from build123d import *
from OCP.BRepFilletAPI import BRepFilletAPI_MakeChamfer

# Parameters (mm, degrees)
SKETCH1_W           = 40
SKETCH1_H           = 30
BOSS_EXTRUDE1_DEPTH = 6
SKETCH2_R           = 1.5
CUT_EXTRUDE1_DEPTH  = 6
FILLET1_R           = 4
SKETCH3_W           = 21
SKETCH3_H           = 21
CUT_EXTRUDE2_DEPTH  = 4
SKETCH6_W           = 5
SKETCH6_H           = 5
CUT_EXTRUDE3_DEPTH  = 2
SKETCH7_W           = 7
SKETCH7_H           = 7
SKETCH7_W_2         = 5
SKETCH7_H_2         = 5
BOSS_EXTRUDE2_DEPTH = 4
CHAMFER1_SIZE       = 4
CHAMFER1_SIZE2      = 6.92820323
CHAMFER2_SIZE       = 5
CHAMFER2_SIZE2      = 2.886751346


with BuildPart() as part:
    # Sketch1 → Boss-Extrude1 (new body)
    with BuildSketch(Plane(origin=(0, 0, 0), x_dir=(1, 0, 0), z_dir=(0, 1, 0))):
        with Locations((20, 15)):
            Rectangle(SKETCH1_W, SKETCH1_H)
    extrude(amount=BOSS_EXTRUDE1_DEPTH)

    # Sketch2 → Cut-Extrude1 (cut)
    with BuildSketch(Plane(origin=(0, 6, 0), x_dir=(1, 0, 0), z_dir=(0, 1, 0))):
        with Locations(Location((5, 5, 0), (0, 0, 270))):
            Circle(SKETCH2_R)
        with Locations(Location((5, 25, 0), (0, 0, 90))):
            Circle(SKETCH2_R)
        with Locations(Location((35, 5, 0), (0, 0, 90))):
            Circle(SKETCH2_R)
        with Locations(Location((35, 25, 0), (0, 0, 270))):
            Circle(SKETCH2_R)
    extrude(amount=-CUT_EXTRUDE1_DEPTH, mode=Mode.SUBTRACT)

    # Fillet1
    fillet1_edges = [part.edges().sort_by_distance(p)[0] for p in [
        (0, 3, -30),
        (40, 3, -30),
        (40, 3, 0),
        (0, 3, 0),
    ]]
    fillet(fillet1_edges, radius=FILLET1_R)

    # Sketch3 → Cut-Extrude2 (cut)
    with BuildSketch(Plane(origin=(0, 6, 0), x_dir=(1, 0, 0), z_dir=(0, 1, 0))):
        with Locations((20, 15)):
            Rectangle(SKETCH3_W, SKETCH3_H)
    extrude(amount=-CUT_EXTRUDE2_DEPTH, mode=Mode.SUBTRACT)

    # Sketch6 → Cut-Extrude3 (cut)
    with BuildSketch(Plane(origin=(0, 2, 0), x_dir=(1, 0, 0), z_dir=(0, 1, 0))):
        with Locations((20, 16)):
            Rectangle(SKETCH6_W, SKETCH6_H)
    extrude(amount=-CUT_EXTRUDE3_DEPTH, mode=Mode.SUBTRACT)

    # Sketch7 → Boss-Extrude2 (add)
    with BuildSketch(Plane(origin=(0, 2, 0), x_dir=(1, 0, 0), z_dir=(0, 1, 0))):
        with Locations((20, 16)):
            Rectangle(SKETCH7_W, SKETCH7_H)
        with Locations((20, 16)):
            Rectangle(SKETCH7_W_2, SKETCH7_H_2, mode=Mode.SUBTRACT)
    extrude(amount=BOSS_EXTRUDE2_DEPTH)

    # Chamfer1: one chamfer whose edges measure the first distance from different faces: ONE call of the kernel's chamfer builder (chamfer() names one face for all edges)
    chamfer1_edges_1 = [part.edges().sort_by_distance(p)[0] for p in [
        (20, 0, -13.5),
    ]]
    chamfer1_side_1 = [part.faces().sort_by_distance(p)[0] for p in [
        (20, 3, -13.5),
    ]]
    chamfer1_edges_2 = [part.edges().sort_by_distance(p)[0] for p in [
        (22.5, 0, -16),
    ]]
    chamfer1_side_2 = [part.faces().sort_by_distance(p)[0] for p in [
        (22.5, 3, -16),
    ]]
    chamfer1_edges_3 = [part.edges().sort_by_distance(p)[0] for p in [
        (20, 0, -18.5),
    ]]
    chamfer1_side_3 = [part.faces().sort_by_distance(p)[0] for p in [
        (20, 3, -18.5),
    ]]
    chamfer1_edges_4 = [part.edges().sort_by_distance(p)[0] for p in [
        (17.5, 0, -16),
    ]]
    chamfer1_side_4 = [part.faces().sort_by_distance(p)[0] for p in [
        (17.5, 3, -16),
    ]]
    chamfer1 = BRepFilletAPI_MakeChamfer(part.part.solid().wrapped)
    for e in chamfer1_edges_1:
        chamfer1.Add(CHAMFER1_SIZE, CHAMFER1_SIZE2, e.wrapped, chamfer1_side_1[0].wrapped)  # the first distance lies on this face
    for e in chamfer1_edges_2:
        chamfer1.Add(CHAMFER1_SIZE, CHAMFER1_SIZE2, e.wrapped, chamfer1_side_2[0].wrapped)  # the first distance lies on this face
    for e in chamfer1_edges_3:
        chamfer1.Add(CHAMFER1_SIZE, CHAMFER1_SIZE2, e.wrapped, chamfer1_side_3[0].wrapped)  # the first distance lies on this face
    for e in chamfer1_edges_4:
        chamfer1.Add(CHAMFER1_SIZE, CHAMFER1_SIZE2, e.wrapped, chamfer1_side_4[0].wrapped)  # the first distance lies on this face
    add(Compound.cast(chamfer1.Shape()), mode=Mode.REPLACE)

    # Chamfer2
    chamfer2_edges = [part.edges().sort_by_distance(p)[0] for p in [
        (16.5, 2, -16),
        (20, 2, -12.5),
        (23.5, 2, -16),
        (20, 2, -19.5),
    ]]
    chamfer2_side = [part.faces().sort_by_distance(p)[0] for p in [
        (20, 2, -4.796984848),
    ]]
    chamfer(chamfer2_edges, length=CHAMFER2_SIZE, length2=CHAMFER2_SIZE2, reference=chamfer2_side[0])


solid = part.part
Model file for the job. Use its own axes, mm. A direction names the side the tool comes from. Coordinates: 2 decimals unless noted, no trailing zeros. Order: outer loops, then holes, each group sorted by start corner. A loop starts at its lowest first (then second) coordinate and runs counter-clockwise, first axis right, second up. Notation, with made-up numbers: (73.25, 65) -> (104.25, 65) arc R21 ccw to (104.25, 85) -> close; hole circle Ø8 at (81.25, 4.25). An arc over 180 degrees is marked (long way). Return JSON: item names as keys, results as strings. Group by question number.
Item 1: Pull direction X, two halves, no side cores. Call faces 5 (the flat face through (20, 0, -5)), 6 (the flat face through (26.78, 1.53, -15.87)), 7 (the cylindrical face through (38.797, 3.042, -1.141)), 8 (the flat face through (20, 4, -25.5)): pulls with the +X half, pulls with the -X half, needs draft (parallel to the pull), parting line crosses it, or undercut.
Item 2: Tool access for faces 1 (the flat face through (20, 3, -30)), 2 (the flat face through (30.5, 4, -15)), 3 (the flat face through (19.87, 1.53, -9.22)), 4 (the flat face through (20, 5, -18.5)): list every direction of +Z, -Z, +X, -X, +Y, -Y with a clear straight run to the whole face (end or side of a thin tool).
Item 3: Saw through at B-B on x = 20. Write the cut outline in (y, z), then the cut area to 3 significant figures.
Item 4: Wall check: line 1 along X through (y, z) = (2.8, -25); line 2 along X through (y, z) = (1.5, -5); line 3 along Z through (x, y) = (11, 4). Give the ranges that are in metal, low to high. Write a range as [from, to].
Item 5: Saw through at C-C on z = -25. Write the cut outline in (x, y), then the cut area to 3 significant figures.
Item 6: Saw through at A-A on x = 5. Write the cut outline in (y, z).
Item 7: Saw through at D-D on y = 3. Write the cut outline in (x, z), then the cut area to 3 significant figures.
Item 8: Flat gauge pin, fed straight in: P1, Ø2, axis at x = 17.5, z = -6, coming from the +Y side. Where does the tip first touch, or does it go through?
Values found:
{
 "1": {"face 5": "needs draft", "face 6": "undercut", "face 7": "pulls with the +X half", "face 8": "undercut"},
 "2": {"face 1": "-Z, +X, -X, +Y, -Y", "face 2": "+Y", "face 3": "-Y", "face 4": "+Y, -Y"},
 "3": {"outline": "(0, -30) -> (6, -30) -> (6, -25.5) -> (2, -25.5) -> (2, -24.5) -> (4.89, -19.5) -> (6, -19.5) -> (6, -18.5) -> (4, -18.5) -> (0, -25.43) -> close; (0, -6.57) -> (4, -13.5) -> (6, -13.5) -> (6, -12.5) -> (4.89, -12.5) -> (2, -7.5) -> (2, -4.5) -> (6, -4.5) -> (6, 0) -> (0, 0) -> close", "area": "80.7 mm2"},
 "4": {"line 1": "x = [0, 3.5], [6.5, 9.5], [30.5, 33.5], [36.5, 40]", "line 2": "x = [0, 3.5], [6.5, 33.5], [36.5, 40]", "line 3": "z = [-30, -25.5], [-4.5, 0]"},
 "5": {"outline": "(0, 0) -> (3.5, 0) -> (3.5, 6) -> (0, 6) -> close; (6.5, 0) -> (10.57, 0) -> (11, 0.25) -> (29, 0.25) -> (29.43, 0) -> (33.5, 0) -> (33.5, 6) -> (30.5, 6) -> (30.5, 2) -> (9.5, 2) -> (9.5, 6) -> (6.5, 6) -> close; (36.5, 0) -> (40, 0) -> (40, 6) -> (36.5, 6) -> close", "area": "115 mm2"},
 "6": {"outline": "(0, -30) -> (6, -30) -> (6, -26.5) -> (0, -26.5) -> close; (0, -23.5) -> (6, -23.5) -> (6, -6.5) -> (0, -6.5) -> close; (0, -3.5) -> (6, -3.5) -> (6, 0) -> (0, 0) -> close"},
 "7": {"outline": "(0, -26) arc R4 ccw to (4, -30) -> (36, -30) arc R4 ccw to (40, -26) -> (40, -4) arc R4 ccw to (36, 0) -> (4, 0) arc R4 ccw to (0, -4) -> close; (13.23, -22.77) -> (26.77, -22.77) -> (26.77, -9.23) -> (13.23, -9.23) -> close; hole circle Ø3 at (5, -25); hole circle Ø3 at (5, -5); hole (9.5, -25.5) -> (30.5, -25.5) -> (30.5, -4.5) -> (9.5, -4.5) -> close; hole (15.77, -20.23) -> (24.23, -20.23) -> (24.23, -11.77) -> (15.77, -11.77) -> close; hole circle Ø3 at (35, -25); hole circle Ø3 at (35, -5)", "area": "829 mm2"},
 "8": {"P1": "stops at y = 2"}
}
